Autodesk Inventor part; units mm, degrees
ref_plane "Work Plane1" through (30, 0, 0) normal (0, -0.5, 0.866) x (1, 0, 0)
ref_plane "YZ Plane" through (0, 0, 0) normal (1, 0, 0) x (0, 1, 0)
ref_plane "XZ Plane" through (0, 0, 0) normal (0, 1, 0) x (-1, 0, 0)
sketch "Sketch1" plane through (0, 0, 0) normal (0, 0, 1) x (1, 0, 0)
  line L0 (-0.19, 0) -> (40, 0)
  line L1 (40, 0) -> (40, 2.5)
  line L2 (40, 2.5) -> (1.6, 2.5)
  line L3 (1.6, 2.5) -> (1.1092, 2.5)
  line L4 (1.1092, 2.5) -> (0, 2.5)
  line L5 (0, 2.5) -> (0, 4.75)
  line L6 (0, 4.75) -> (-2.75, 4.75)
  line L7 (-2.75, 4.75) -> (-2.75, 1.7321)
  line L8 (-2.75, 1.7321) -> (-1.19, 1.7321)
  line L9 (-1.19, 1.7321) -> (-0.19, 0)
  line L10 (-11.3, 0) -> (48.55, 0)
  line L11 (0, -0.95) -> (0, 5.7)
  line L12 (1.6, 2.5) -> (0, 2.5) construction
  dimension "d0" = 38.4
  dimension "d1" = 0.4908
  dimension "d2" = 2.75
  dimension "d3" = 1.56
  dimension "d4" = 60
  dimension "d5" = 5
  dimension "d6" = 5
  dimension "d7" = 3.4641
  dimension "d8" = 9.5
  dimension "d19" = 40
revolve "Body" add sketch "Sketch1" angle 360 about axis through (-0.19, 0, 0) along (1, 0, 0)
sketch "Sketch2" plane through (-2.75, 0, 0) normal (-1, 0, 0) x (0, 0, 1)
  circle A0 centre (0, 0) radius 1.7321
  line L0 (0, -6.65) -> (0, 6.65)
  line L1 (-6.65, 0) -> (6.65, 0)
  line L2 (1.7321, 0) -> (0.866, -1.5)
  line L3 (0.866, -1.5) -> (-0.866, -1.5)
  line L4 (-0.866, -1.5) -> (-1.7321, 0)
  line L5 (-1.7321, 0) -> (-0.866, 1.5)
  line L6 (-0.866, 1.5) -> (0.866, 1.5)
  line L7 (0.866, 1.5) -> (1.7321, 0)
extrude "Slot" add sketch "Sketch2" against normal up to next contours L7 A0 | A0 L2 | L6 L0 A0 | A0 L0 L3 | L0 L6 A0 | A0 L3 L0 | L4 A0 | A0 L5
fillet "Fillet1" radius 2.375 1 edges at (-2.75, -4.75, 0)
thread "Thread"
chamfer "Chamfer1" distance 0.4908 distance2 0.4908 1 edges at (40, -2.5, 0) measured on face at (40, 0.9945, 0.5526)
fillet "Fillet2" radius 0.2 1 edges at (0, -2.5, 0)
ref_plane "Work Plane1" through (30, 0, 0) normal (0, -0.5, 0.866) x (1, 0, 0)
equation "\"d0\" = GEL"
equation "\"d1\" = GAL"
equation "\"d2\" = KOH"
equation "\"d3\" = INTI"
equation "\"d5\" = GD"
equation "\"d6\" = BDM"
equation "\"d7\" = 1.1547 * SW"
equation "\"d8\" = KOD"
equation "\"d19\" = NLG"
equation "\"d16\" = RR"
equation "\"d12\" = GEL"
equation "\"d14\" = -0.5 * SPD + 0.5 * GD"
equation "\"d15\" = GUL"
equation "\"d29\" = R"
equation "\"GD\" = NND"
equation "\"NLG\" = 40"
equation "\"GEL\" = 38.4"
equation "\"KOD\" = 9.5"
equation "\"KOH\" = 2.75"
equation "\"INTI\" = 1.56"
equation "\"GAL\" = 0.61345 * PTC"
equation "\"GUL\" = 0.61345 * PTC"
equation "\"BDM\" = NND"
equation "\"SW\" = 3"
equation "\"RR\" = 2.375"
equation "\"SPD\" = 4.01848"
equation "\"d28\" = R"
equation "\"R\" = 0.2"
equation "\"TOA\" = 30deg"
equation "\"THREADDIA\" = 5"
equation "\"KOD1\" = KOD - 2 * RR"
equation "\"PTC\" = 0.8"
equation "\"NND\" = 5"
equation "\"E0\" = 1.155 * SW"
equation "\"GD1\" = THREADDIA - 1.2269 * PTC"
properties part number "ANSI B18.3.4M - M5 x 0.8 x 40" material "Steel, Mild"
Geometry check sheet. Reference: the model listing, model coordinates, mm. A direction names the side the tool comes from. Coordinates: 2 decimals unless noted, no trailing zeros. Order: outer loops, then holes, each group sorted by start corner. A loop starts at its lowest first (then second) coordinate and runs counter-clockwise, first axis right, second up. Notation, with made-up numbers: (42.25, -12.5) -> (72.25, -12.5) arc R14 cw to (72.25, 12.5) -> close; hole circle Ø8 at (68.25, -2.75). An arc over 180 degrees is marked (long way). Use a Markdown table: item, result. Add a question column.
1. Mould release check, pull along Z, two halves, no side actions. Record for faces 1 (the face through (-0.19, 2.192, 4.214)), 2 (the face through (0, 2.04, -2.04)), 3 (the face through (-1.915, -0.74, 1.305)): pulls with the +Z half, pulls with the -Z half, needs draft (parallel to the pull), parting line crosses it, or undercut.
2. Set-up check for faces 4 (the face through (-2, 1.5, 0)), 5 (the face through (-2.75, -2, 0)), 6 (the face through (19.58, -0.54, 2.44)): record each of +Z, -Z, +X, -X, +Y, -Y from which the full face is reachable in a straight line by a thin tool's end or side.
3. Cross-section at A-A (x = 2). Enter the section's corners in (y, z), and give its area (3 significant figures).
4. Material ranges on L1, parallel to Z at x = 14.5, y = 0; L2, parallel to Y at x = 28, z = 0.75; L3, parallel to Y at x = 11.5, z = -1.5, recorded low to high.
5. Go/stop test with flat-tipped pins: pin 1 Ø2 at (x, z) = (18, 1.5) entering from +Y; pin 2 Ø0.5 at (x, z) = (-2, 0) entering from +Y; pin 3 Ø1.5 at (x, z) = (16, -0.5) entering from +Y. Record where each tip stops, or that it passes through.
Filled sheet:
| question | item | result |
|---|---|---|
| 1 | face 1 | parting line crosses it |
| 1 | face 2 | needs draft |
| 1 | face 3 | undercut |
| 2 | face 4 | -X |
| 2 | face 5 | +Z, -Z, -X, +Y, -Y |
| 2 | face 6 | +X |
| 3 | outline | circle Ø5 at (0, 0) |
| 3 | area | 19.6 mm2 |
| 4 | L1 | -2.5 to 2.5 |
| 4 | L2 | -2.38 to 2.38 |
| 4 | L3 | -2 to 2 |
| 5 | pin 1 | y = 2.45 |
| 5 | pin 2 | y = 4.31 |
| 5 | pin 3 | y = 2.5 |
